from build123d import *

# Parameters (mm, degrees)
F1_R     = 2.5
F2_DEPTH = 8
F0_W     = 20
F0_H     = 20
F3_DEPTH = 8


with BuildPart() as f2:
    # F1 (on face) → F2 (new body)
    with BuildSketch(Plane.XY):
        with Locations((-6, -5)):
            Circle(F1_R)
    extrude(amount=F2_DEPTH)

    # F0 (on Top) → F3 (join)
    with BuildSketch(Plane.XY):
        Rectangle(F0_W, F0_H)
    extrude(amount=-F3_DEPTH)


solid = f2.part
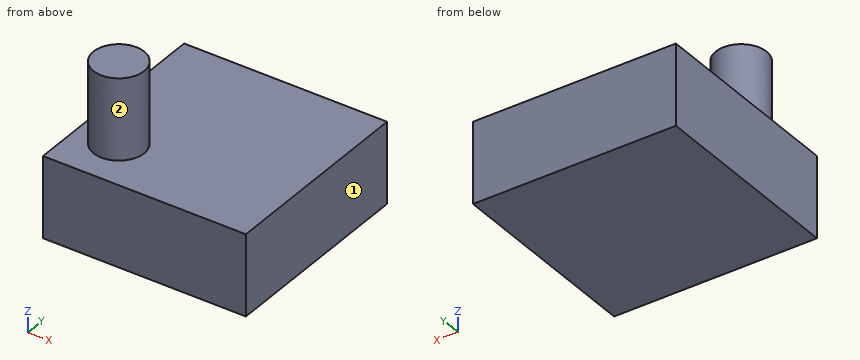
Here's how the part is built. I have some questions about the finished solid (model axes, mm). Face numbers are marked on the shaded views. A direction names the side the tool comes from. Round coordinates to 2 decimals unless told otherwise and drop trailing zeros. Order: outer loops, then holes, each group sorted by start corner. A loop starts at its lowest first (then second) coordinate and runs counter-clockwise, first axis right, second up. Notation, with made-up numbers: (-13, -10.5) -> (13, -10.5) arc R27 cw to (13, 11.5) -> close; hole circle Ø1 at (1, 8.25). An arc over 180 degrees is marked (long way). Use CSV: the item, a comma, the result in double quotes.
1. I want a section at A-A on x = -6. List the corners of the cut face in (y, z) for me.
Recorded:
outline,"(-10, -8) -> (10, -8) -> (10, 0) -> (-2.5, 0) -> (-2.5, 8) -> (-7.5, 8) -> (-7.5, 0) -> (-10, 0) -> close"
2. Which directions (+Z, -Z, +X, -X, +Y, -Y) give clear straight access to the entire face, cutting with the end or side of a thin tool? Please do the marked faces 1 and 2.
Recorded:
face 1,"+Z, -Z, +X, +Y, -Y"
face 2,"+Z"
3. I'm going to push flat-ended pins straight in: P1, Ø10, axis at x = 6.5, y = 7, coming from the +Z side; P2, Ø1.5, axis at y = -3.5, z = 1, coming from the -X side; P3, Ø6, axis at x = -3.5, z = 4.5, coming from the +Y side. Where does each tip first touch, or does it pass through?
Recorded:
P1,"stops at z = 0"
P2,"stops at x = -8.38"
P3,"stops at y = -2.5"
4. I need wall thicknesses on line 1 along Z through (x, y) = (7.25, -9); line 2 along X through (y, z) = (-4, 3.25); line 3 along Y through (x, z) = (-8, 2.5). Which ranges of each line are inside material? Lowest first, please.
Recorded:
line 1,"z = -8 to 0"
line 2,"x = -8.29 to -3.71"
line 3,"y = -6.5 to -3.5"
5. I want a section at D-D on x = -2. List the corners of the cut face in (y, z) for me, and give its area (3 significant figures).
Recorded:
outline,"(-10, -8) -> (10, -8) -> (10, 0) -> (-10, 0) -> close"
area,"160 mm2"
6. I want a section at C-C on z = 3.25. List the corners of the cut face in (x, y) for me, and give its area (3 significant figures).
Recorded:
outline,"circle Ø5 at (-6, -5)"
area,"19.6 mm2"
7. I want a section at B-B on y = -5. List the corners of the cut face in (x, z) for me, and give its area (3 significant figures).
Recorded:
outline,"(-10, -8) -> (10, -8) -> (10, 0) -> (-3.5, 0) -> (-3.5, 8) -> (-8.5, 8) -> (-8.5, 0) -> (-10, 0) -> close"
area,"200 mm2"
